from build123d import *

# Parameters (mm, degrees)
BOSS_EXTRUDE1_DEPTH      = 1.75
BOSS_EXTRUDE1_DEPTH_BACK = 1.75
SKETCH1_R                = 5
SKETCH1_R_2              = 3
BOSS_EXTRUDE4_DEPTH      = 2
BOSS_EXTRUDE4_DEPTH_BACK = 2
BOSS_EXTRUDE2_START      = 2
SKETCH1_3_R              = 3.4999999999999996
SKETCH1_3_R_2            = 1.5000000000000024
BOSS_EXTRUDE2_DEPTH      = 3
BOSS_EXTRUDE3_START      = -5
SKETCH1_4_R              = 3.4999999999999996
SKETCH1_4_R_2            = 1.5000000000000024
BOSS_EXTRUDE3_DEPTH      = 3
FILLET2_R                = 2


with BuildPart() as part:
    # Sketch1 → Boss-Extrude1 (new, two sides: drawn at the far end of the back side and taken through both)
    # profile 1 of 3: a face of its own
    with BuildSketch(Plane(origin=(0, 0, 0), x_dir=(0, 0, -1), z_dir=(1, 0, 0)).offset(-BOSS_EXTRUDE1_DEPTH_BACK)):
        with BuildLine():
            Line((4.128289444917901, 2.820855589883948), (-2.446958304851689, 12.443654424549113))
            Line((-2.4469583048516905, 12.443654424549113), (-9.553041695148336, 8.340955266277398))
            Line((-9.553041695148337, 8.340955266277398), (-4.507077323705776, -2.1647757385320965))
            ThreePointArc((-4.507077323705776, -2.1647757385320965), (-2.500000000000005, 4.33012701892219), (4.128289444917895, 2.8208555898839442))
        make_face()
    # profile 2 of 3: a face of its own
    with BuildSketch(Plane(origin=(0, 0, 0), x_dir=(0, 0, -1), z_dir=(1, 0, 0)).offset(-BOSS_EXTRUDE1_DEPTH_BACK)):
        Circle(SKETCH1_R)
        Circle(SKETCH1_R_2, mode=Mode.SUBTRACT)
    # profile 3 of 3: a face of its own
    with BuildSketch(Plane(origin=(0, 0, 0), x_dir=(0, 0, -1), z_dir=(1, 0, 0)).offset(-BOSS_EXTRUDE1_DEPTH_BACK)):
        Polygon((-2.446958304851689, 12.443654424549113), (-4.710146578566388, 15.755804219010134), (-11.289853421433653, 11.957008702091882), (-9.553041695148337, 8.340955266277398), align=None)
    extrude(amount=BOSS_EXTRUDE1_DEPTH + BOSS_EXTRUDE1_DEPTH_BACK)

    # Sketch1<5> → Boss-Extrude4 (add, two sides: drawn at the far end of the back side and taken through both)
    with BuildSketch(Plane(origin=(0, 0, 0), x_dir=(0, 0, -1), z_dir=(1, 0, 0)).offset(-BOSS_EXTRUDE4_DEPTH_BACK)):
        Polygon((-2.446958304851689, 12.443654424549113), (-4.710146578566388, 15.755804219010134), (-11.289853421433653, 11.957008702091882), (-9.553041695148337, 8.340955266277398), align=None)
    extrude(amount=BOSS_EXTRUDE4_DEPTH + BOSS_EXTRUDE4_DEPTH_BACK)

    # Sketch1<3> → Boss-Extrude2 (add)
    # profile 1 of 3: a face of its own
    with BuildSketch(Plane(origin=(0, 0, 0), x_dir=(0, 0, -1), z_dir=(1, 0, 0)).offset(BOSS_EXTRUDE2_START)):
        Polygon((-2.446958304851689, 12.443654424549113), (-4.710146578566388, 15.755804219010134), (-11.289853421433653, 11.957008702091882), (-9.553041695148337, 8.340955266277398), align=None)
    # profile 2 of 3: a face of its own
    with BuildSketch(Plane(origin=(0, 0, 0), x_dir=(0, 0, -1), z_dir=(1, 0, 0)).offset(BOSS_EXTRUDE2_START)):
        with BuildLine():
            Line((-4.710146578566388, 15.755804219010134), (-7.0101973885575, 19.12190190785064))
            ThreePointArc((-7.010197388557501, 19.12190190785064), (-6.556027127797799, 18.18066906268114), (-6.400000000000027, 17.147302994931877))
            ThreePointArc((-6.400000000000027, 17.147302994931877), (-9.122934829978606, 13.734654504164101), (-13.054954126594069, 15.63195997795941))
            Line((-13.054954126594073, 15.631959977959408), (-11.289853421433653, 11.957008702091882))
            Line((-11.289853421433653, 11.957008702091882), (-4.7101465785663885, 15.755804219010134))
        make_face()
    # profile 3 of 3: a face of its own
    with BuildSketch(Plane(origin=(0, 0, 0), x_dir=(0, 0, -1), z_dir=(1, 0, 0)).offset(BOSS_EXTRUDE2_START)):
        with Locations((-9.900000000000027, 17.147302994931877)):
            Circle(SKETCH1_3_R)
        with Locations((-9.900000000000027, 17.147302994931877)):
            Circle(SKETCH1_3_R_2, mode=Mode.SUBTRACT)
    extrude(amount=BOSS_EXTRUDE2_DEPTH)

    # Sketch1<4> → Boss-Extrude3 (add)
    # profile 1 of 3: a face of its own
    with BuildSketch(Plane(origin=(0, 0, 0), x_dir=(0, 0, -1), z_dir=(1, 0, 0)).offset(BOSS_EXTRUDE3_START)):
        with BuildLine():
            Line((-4.710146578566388, 15.755804219010134), (-7.0101973885575, 19.12190190785064))
            ThreePointArc((-7.010197388557501, 19.12190190785064), (-6.556027127797799, 18.18066906268114), (-6.400000000000027, 17.147302994931877))
            ThreePointArc((-6.400000000000027, 17.147302994931877), (-9.122934829978606, 13.734654504164101), (-13.054954126594069, 15.63195997795941))
            Line((-13.054954126594073, 15.631959977959408), (-11.289853421433653, 11.957008702091882))
            Line((-11.289853421433653, 11.957008702091882), (-4.7101465785663885, 15.755804219010134))
        make_face()
    # profile 2 of 3: a face of its own
    with BuildSketch(Plane(origin=(0, 0, 0), x_dir=(0, 0, -1), z_dir=(1, 0, 0)).offset(BOSS_EXTRUDE3_START)):
        Polygon((-2.446958304851689, 12.443654424549113), (-4.710146578566388, 15.755804219010134), (-11.289853421433653, 11.957008702091882), (-9.553041695148337, 8.340955266277398), align=None)
    # profile 3 of 3: a face of its own
    with BuildSketch(Plane(origin=(0, 0, 0), x_dir=(0, 0, -1), z_dir=(1, 0, 0)).offset(BOSS_EXTRUDE3_START)):
        with Locations((-9.900000000000027, 17.147302994931877)):
            Circle(SKETCH1_4_R)
        with Locations((-9.900000000000027, 17.147302994931877)):
            Circle(SKETCH1_4_R_2, mode=Mode.SUBTRACT)
    extrude(amount=BOSS_EXTRUDE3_DEPTH)

    # Fillet2
    fillet2_edges = [part.edges().sort_by_distance(p)[0] for p in [
        (-3.375, 12.443654424549113, 2.4469583048516905),
        (-3.375, 8.340955266277398, 9.553041695148337),
        (3.375, 12.443654424549113, 2.44695830485169),
        (3.375, 8.340955266277398, 9.553041695148337),
    ]]
    fillet(fillet2_edges, radius=FILLET2_R)


solid = part.part
Input: part model. Units: mm. Frame: model coordinates. A direction names the side the tool comes from. Coordinates: 2 decimals unless noted, no trailing zeros. Loops run counter-clockwise (first coordinate to the right, second up) from the corner with the lowest first, then second, coordinate; pieces in that order, holes last. Notation, with made-up numbers: (58.5, -14) - (106.5, -14) arc R33 cw to (106.5, 17) - close; hole circle Ø5 at (-21.5, -24.75). An arc over 180 degrees is marked (long way). Answer in a Markdown table with one row per item. Add a question column.
Item 1: Line query: line 1 along X through (y, z) = (9.75, 3); line 2 along Y through (x, z) = (0, 0); line 3 along Z through (x, y) = (4.5, 17.25). Output: solid intervals per line, ascending. Write a range as [from, to].
Item 2: Contact query for flat-ended pins moving along their axis: P1, Ø7.5, axis at y = 3.5, z = 0.5, coming from the +X side; P2, Ø2.5, axis at y = 17.15, z = 9.9, coming from the +X side; P3, Ø4, axis at x = -0.5, y = 10, coming from the -Z side; P4, Ø4, axis at x = -1, y = 13.5, coming from the -Z side. Output: stop coordinate, or through.
Item 3: Access query for faces 4 (the cylindrical face through (3.35, 12.68, 3.36)), 5 (the cylindrical face through (3.35, 9.25, 9.3)), 6 (the cylindrical face through (-3.4, 9.25, 9.3)), 7 (the flat face through (-2, 15, 9)). Directions: +Z, -Z, +X, -X, +Y, -Y. A direction counts if a zero-diameter tool reaches every point of the face in a straight line with its end or side. Return the directions, or none.
Item 4: Mould query, pull axis Y, two halves, no side actions, for faces 1 (the flat face through (3.35, 10.38, 6.02)), 2 (the cylindrical face through (-3.52, 18.41, 9.09)), 3 (the flat face through (1.75, 5, 3)). Classes: released by +Y, released by -Y, zero draft, split by the parting line, or undercut.
Item 5: Section query A-A on y = -2.5. Return the cut outline in (x, z).
Item 6: Section query D-D on z = 0. Return the cut outline in (x, y), then the cut area to 3 significant figures.
Item 7: Section query C-C on x = -1. Return the cut outline in (y, z).
Item 8: Section query B-B on z = 9.9. Return the cut outline in (x, y).
Recorded:
| question | item | result |
|---|---|---|
| 1 | line 1 | [-1.75, 1.75] |
| 1 | line 2 | [-5, -3], [3, 8.86] |
| 1 | line 3 | [5.73, 8.4], [11.4, 13.4] |
| 2 | P1 | x = 1.75 |
| 2 | P2 | through |
| 2 | P3 | z = -0.59 |
| 2 | P4 | z = 1.8 |
| 3 | face 4 | -Z, +X |
| 3 | face 5 | +X, -Y |
| 3 | face 6 | -X, -Y |
| 3 | face 7 | +Z, +Y |
| 4 | face 1 | released by -Y |
| 4 | face 2 | undercut |
| 4 | face 3 | zero draft |
| 5 | outline | (-1.75, -4.33) - (1.75, -4.33) - (1.75, -1.66) - (-1.75, -1.66) - close; (-1.75, 1.66) - (1.75, 1.66) - (1.75, 4.33) - (-1.75, 4.33) - close |
| 6 | outline | (-1.75, -5) - (1.75, -5) - (1.75, -3) - (-1.75, -3) - close; (-1.75, 3) - (1.75, 3) - (1.75, 8.86) - (-1.75, 8.86) - close |
| 6 | area | 27.5 mm^2 |
| 7 | outline | (-2.16, 4.51) arc R5 ccw (long way) to (2.82, -4.13) - (15.76, 4.71) - (11.96, 11.29) - close; hole circle Ø6 at (0, 0) |
| 8 | outline | (-5, 9.56) - (-1.75, 9.56) - (-1.75, 9.06) - (1.75, 9.06) - (1.75, 9.56) - (5, 9.56) - (5, 15.65) - (2, 15.65) - (2, 12.76) - (-2, 12.76) - (-2, 15.65) - (-5, 15.65) - close; (-5, 18.65) - (-2, 18.65) - (-2, 20.65) - (-5, 20.65) - close; (2, 18.65) - (5, 18.65) - (5, 20.65) - (2, 20.65) - close |
